Check sheet for the drawn part. Datum: minimum x, y, z corner. Units: mm. A direction names the side the tool comes from. Coordinates: 2 decimals unless noted, no trailing zeros. Order: outer loops, then holes, each group sorted by start corner. A loop starts at its lowest first (then second) coordinate and runs counter-clockwise, first axis right, second up. Notation, with made-up numbers: M 41.25,-17.75 L 55.25,-17.75 A15 ccw 55.25,-13.75 Z; hole C -6,74 d10. An arc over 180 degrees is marked long. Return JSON: item names as keys, results as strings. Group by question number.
Q1. Mould release check, pull along Z, two halves, no side actions. Record for the marked faces 1, 2 and 3: pulls with the +Z half, pulls with the -Z half, needs draft (parallel to the pull), parting line crosses it, or undercut.
Q2. Section check B-B, the plane y = 5.65. Enter the section's corners in (x, z), then the cut area to 4 significant figures.
Q3. Go/stop test with flat-tipped pins: pin 1 Ø6 at (x, z) = (20.5, 23) entering from +Y; pin 2 Ø10 at (y, z) = (25.5, 16.5) entering from -X; pin 3 Ø0.9 at (x, y) = (6.5, 5.5) entering from +Z. Record where each tip stops, or that it passes through.
Q4. Section check A-A, the plane x = 21.15. Enter the section's corners in (y, z).
Q5. Section check D-D, the plane y = 12.5. Enter the section's corners in (x, z), then the cut area to 3 significant figures.
Q6. Thickness scan on probe 1 along Y at (x, z) = (5.65, 37.75); probe 2 along Y at (x, z) = (5, 37). Record the ranges inside material, lowest first.
Q7. Access from +Z, -Z, +X, -X, +Y, -Y to the whole of each face (thin tool, end or side, straight path). Record for the marked faces 4, 5, 6, 7 and 8.
Q8. Section check C-C, the plane z = 8.5. Enter the section's corners in (x, y).
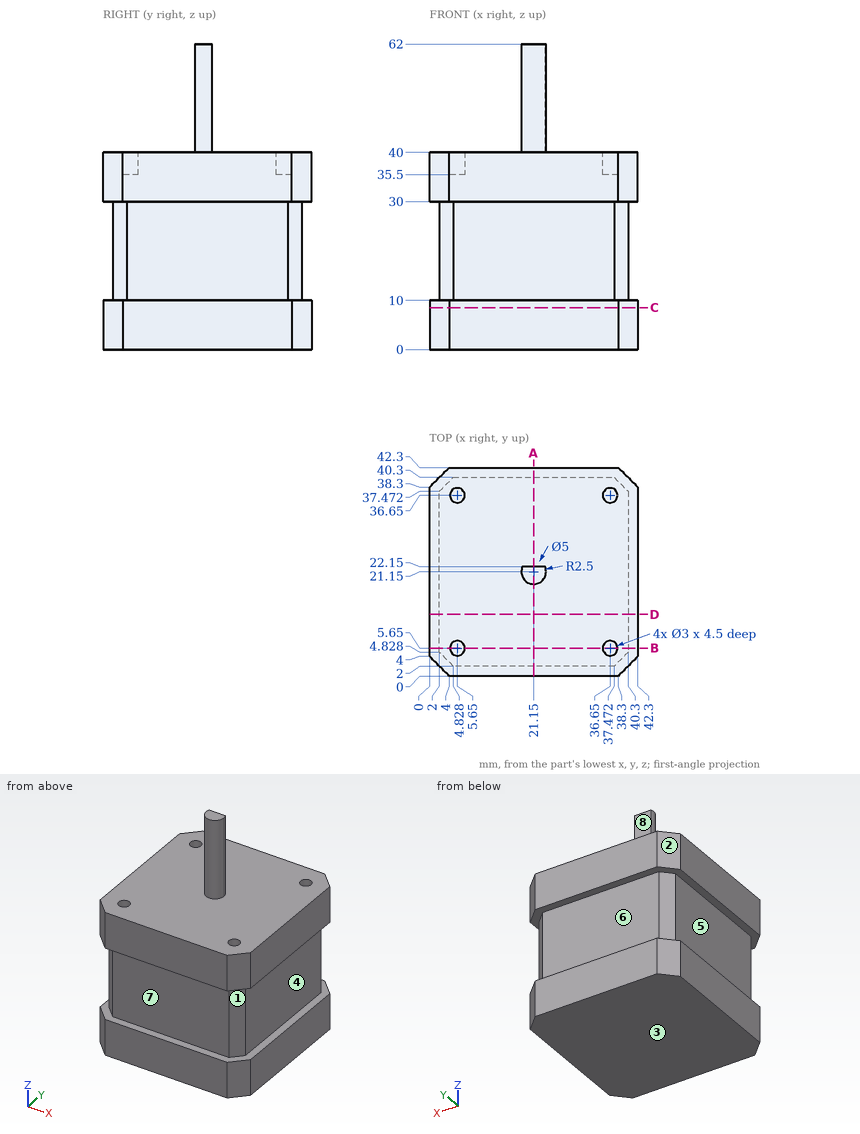
Numbers:
{
 "1": {"face 1": "undercut", "face 2": "needs draft", "face 3": "pulls with the -Z half"},
 "2": {"outline": "M 0,0 L 42.3,0 L 42.3,10 L 40.3,10 L 40.3,30 L 42.3,30 L 42.3,40 L 38.15,40 L 38.15,35.5 L 35.15,35.5 L 35.15,40 L 7.15,40 L 7.15,35.5 L 4.15,35.5 L 4.15,40 L 0,40 L 0,30 L 2,30 L 2,10 L 0,10 Z", "area": "1,585 mm2"},
 "3": {"pin 1": "stops at y = 40.3", "pin 2": "stops at x = 2", "pin 3": "stops at z = 35.5"},
 "4": {"outline": "M 0,0 L 42.3,0 L 42.3,10 L 40.3,10 L 40.3,30 L 42.3,30 L 42.3,40 L 22.15,40 L 22.15,62 L 18.65,62 L 18.65,40 L 0,40 L 0,30 L 2,30 L 2,10 L 0,10 Z"},
 "5": {"outline": "M 0,0 L 42.3,0 L 42.3,10 L 40.3,10 L 40.3,30 L 42.3,30 L 42.3,40 L 0,40 L 0,30 L 2,30 L 2,10 L 0,10 Z", "area": "1,610 mm2"},
 "6": {"probe 1": "y = 0 to 4.15, 7.15 to 35.15, 38.15 to 42.3", "probe 2": "y = 0 to 4.3, 7 to 35.3, 38 to 42.3"},
 "7": {"face 4": "+X, +Y, -Y", "face 5": "-X, +Y, -Y", "face 6": "+X, -X, +Y", "face 7": "+X, -X, -Y", "face 8": "+Z, +X, -X, +Y"},
 "8": {"outline": "M 0,4 L 4,0 L 38.3,0 L 42.3,4 L 42.3,38.3 L 38.3,42.3 L 4,42.3 L 0,38.3 Z"}
}
